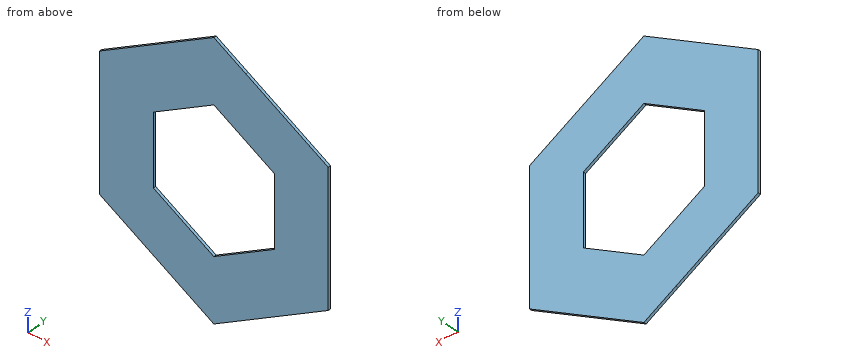
```python
from build123d import *

# Parameters (mm, degrees)
RESSALTO_EXTRUS_O1_DEPTH = 1
CORTE_EXTRUS_O1_DEPTH    = 67.638154236


with BuildPart() as part:
    # Esboço1 → Ressalto-extrusão1 (new body)
    with BuildSketch(Plane(origin=(0, 0, 0), x_dir=(1, 0, 0), z_dir=(0, 1, 0))):
        Polygon((-43.62, 11.068078609), (-43.62, 25.184018742), (-12.224762753, 43.310067418), (0, 50.368037484), (31.395237247, 32.241988808), (43.62, 25.184018742), (43.62, -11.068078609), (43.62, -25.184018742), (12.224762753, -43.310067418), (0, -50.368037484), (-31.395237247, -32.241988808), (-43.62, -25.184018742), align=None)
    extrude(amount=RESSALTO_EXTRUS_O1_DEPTH)

    # Esboço2 → Corte-extrusão1 (cut, through all)
    with BuildSketch(Plane.XZ):
        Polygon((23.09165742, 13.331974628), (0, 26.663949255), (-23.09165742, 13.331974628), (-23.09165742, -13.331974628), (0, -26.663949255), (23.09165742, -13.331974628), align=None)
    extrude(amount=-CORTE_EXTRUS_O1_DEPTH, mode=Mode.SUBTRACT)


solid = part.part
```
Geometry: final body of the model. Coordinates: model frame, mm. Coordinates: 2 decimals unless noted, no trailing zeros. Write each loop counter-clockwise with the first axis right and the second up, starting at its lowest first coordinate (ties: lowest second). Pieces come first, ordered by that corner, then holes. Notation, with made-up numbers: M 37,76.25 L 55,76.25 A27 cw 55,102.25 Z; hole C 5,-18.75 d2. An arc over 180 degrees is marked long. Answer as CSV lines item,"result". Start each with the question number.
Q1. Cut plane A-A on z = 1. Return the cut outline in (x, y), then the cut area to 3 significant figures.
Q2. Cut plane D-D on x = 27.5. Return the cut outline in (y, z).
Q3. Cut plane C-C on x = 16. Return the cut outline in (y, z).
Q4. Line query: line 1 (X direction, y = 0.15, z = -17.5); line 2 (Z direction, x = -9.5, y = 0.5); line 3 (X direction, y = 0.65, z = 5.5). Output: solid intervals per line, ascending. Write a range as from..to.
Q5. Cut plane B-B on y = 0.6. Return the cut outline in (x, z), then the cut area to 3 significant figures.
Findings below:
1,outline,"M -43.62,0 L -23.09,0 L -23.09,1 L -43.62,1 Z; M 23.09,0 L 43.62,0 L 43.62,1 L 23.09,1 Z"
1,area,"41.1 mm2"
2,outline,"M 0,-34.49 L 1,-34.49 L 1,34.49 L 0,34.49 Z"
3,outline,"M 0,-41.13 L 1,-41.13 L 1,-17.43 L 0,-17.43 Z; M 0,17.43 L 1,17.43 L 1,41.13 L 0,41.13 Z"
4,line 1,"x = -43.62..-15.87, 15.87..43.62"
4,line 2,"z = -44.88..-21.18, 21.18..44.88"
4,line 3,"x = -43.62..-23.09, 23.09..43.62"
5,outline,"M -43.62,-25.18 L 0,-50.37 L 43.62,-25.18 L 43.62,25.18 L 0,50.37 L -43.62,25.18 Z; hole M -23.09,-13.33 L 0,-26.66 L 23.09,-13.33 L 23.09,13.33 L 0,26.66 L -23.09,13.33 Z"
5,area,"4,740 mm2"
